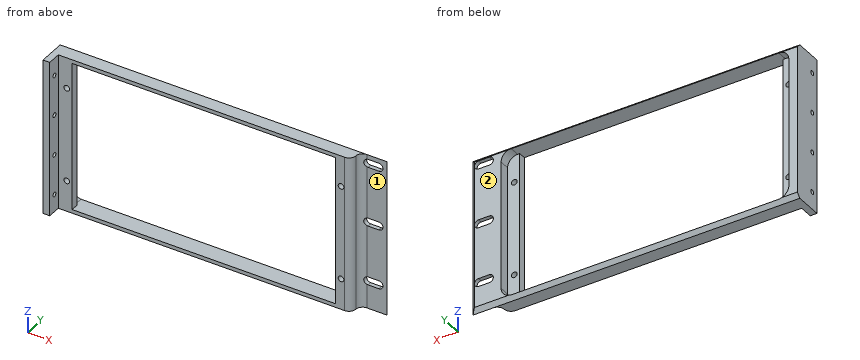
from build123d import *

# Parameters (mm, degrees)
SKETCH1_W                        = 242.5
SKETCH1_H                        = 116
BOSS_EXTRUDE1_DEPTH              = 13
CUT_EXTRUDE1_DEPTH               = 7.6
F_1_8_27_NPSM_TAPPED_HOLE1_D     = 5
F_1_8_27_NPSM_TAPPED_HOLE1_DEPTH = 22.99
F_1_8_27_NPSM_TAPPED_HOLE1_TIP   = 1.502151548
SKETCH6_W                        = 195.5
SKETCH6_H                        = 110.5
CUT_EXTRUDE2_DEPTH               = 143.098592533
SKETCH32_W                       = 20
SKETCH32_H                       = 116
CUT_EXTRUDE10_DEPTH              = 10
FILLET1_START                    = -59
FILLET1_DEPTH                    = 118
FILLET1_START_2                  = -58
FILLET1_2_DEPTH                  = 116
CHAMFER1_SIZE                    = 3
SKETCH36_W                       = 5
SKETCH36_H                       = 116
BOSS_EXTRUDE2_DEPTH              = 10
M5X0_8_TAPPED_HOLE1_D            = 4.2
M5X0_8_TAPPED_HOLE1_DEPTH        = 12.4
M5X0_8_TAPPED_HOLE1_TIP          = 1.2618073
M4X0_7_TAPPED_HOLE1_D            = 3.3
CUT_EXTRUDE11_DEPTH              = 144.747173885


with BuildPart() as part:
    # Sketch1 → Boss-Extrude1 (new body)
    with BuildSketch(Plane(origin=(0, 0, 0), x_dir=(1, 0, 0), z_dir=(0, 1, 0))):
        with Locations((8.25, 0)):
            Rectangle(SKETCH1_W, SKETCH1_H)
    extrude(amount=BOSS_EXTRUDE1_DEPTH)

    # Sketch2 → Cut-Extrude1 (cut)
    with BuildSketch(Plane(origin=(0, 13, 0), x_dir=(1, 0, 0), z_dir=(0, 1, 0))):
        with BuildLine():
            Line((-99.25, 55.25), (99.25, 55.25))
            ThreePointArc((99.25, 55.25), (104.553300859, 53.053300859), (106.75, 47.75))
            Line((106.75, 47.75), (106.75, -47.75))
            ThreePointArc((106.75, -47.75), (104.553300859, -53.053300859), (99.25, -55.25))
            Line((99.25, -55.25), (-99.25, -55.25))
            ThreePointArc((-99.25, -55.25), (-104.553300859, -53.053300859), (-106.75, -47.75))
            Line((-106.75, -47.75), (-106.75, 47.75))
            ThreePointArc((-106.75, 47.75), (-104.553300859, 53.053300859), (-99.25, 55.25))
        make_face()
    extrude(amount=-CUT_EXTRUDE1_DEPTH, mode=Mode.SUBTRACT)

    # 1/8-27 NPSM Tapped Hole1
    with Locations(Plane(origin=(0, 5.4, 0), x_dir=(1, 0, 0), z_dir=(0, 1, 0))):
        with Locations((-74.86, 30.93), (51.34, 30.93), (51.34, -34.72), (-74.86, -34.72)):
            Hole(F_1_8_27_NPSM_TAPPED_HOLE1_D / 2, depth=F_1_8_27_NPSM_TAPPED_HOLE1_DEPTH)
            with Locations((0, 0, -(F_1_8_27_NPSM_TAPPED_HOLE1_DEPTH + F_1_8_27_NPSM_TAPPED_HOLE1_TIP / 2))):  # 118° drill point
                Cone(0, F_1_8_27_NPSM_TAPPED_HOLE1_D / 2, F_1_8_27_NPSM_TAPPED_HOLE1_TIP, mode=Mode.SUBTRACT)

    # Sketch6 → Cut-Extrude2 (cut, through all)
    with BuildSketch(Plane(origin=(0, 5.4, 0), x_dir=(1, 0, 0), z_dir=(0, 1, 0))):
        Rectangle(SKETCH6_W, SKETCH6_H)
    extrude(amount=-CUT_EXTRUDE2_DEPTH, mode=Mode.SUBTRACT)

    # Sketch32 → Cut-Extrude10 (cut)
    with BuildSketch(Plane.XZ):
        with Locations((119.5, 0)):
            Rectangle(SKETCH32_W, SKETCH32_H)
    extrude(amount=-CUT_EXTRUDE10_DEPTH, mode=Mode.SUBTRACT)

    # Fillet1: read off the stored shape, not the designer's step
    # Fillet1 outline → Fillet1 (cut)
    with BuildSketch(Plane.XY.offset(FILLET1_START)):
        with BuildLine():
            Line((109.5, 0), (109.5, 5))
            ThreePointArc((109.5, 5), (108.035533906, 1.464466094), (104.5, 0))
            Line((104.5, 0), (109.5, 0))
        make_face()
    extrude(amount=FILLET1_DEPTH, mode=Mode.SUBTRACT)

    # Fillet1 2 outline → Fillet1 2 (add)
    with BuildSketch(Plane.XY.offset(FILLET1_START_2)):
        with BuildLine():
            ThreePointArc((109.5, 5), (110.964466094, 8.535533906), (114.5, 10))
            Line((114.5, 10), (109.5, 10))
            Line((109.5, 10), (109.5, 5))
        make_face()
    extrude(amount=FILLET1_2_DEPTH)

    # Chamfer1
    # the kernel refuses this chamfer: 3 mm, written as the material it takes off along each edge
    with BuildSketch(Plane(origin=(137.215048964, 13, 58), x_dir=(0, 0, -1), z_dir=(-1, 0, 0))) as chamfer1_piece_1:
        Polygon((CHAMFER1_SIZE, 0), (0, CHAMFER1_SIZE), (0, 0), align=None)
    extrude(amount=257.930097928, mode=Mode.SUBTRACT)
    with BuildSketch(Plane(origin=(129.5, 13, -65.715048964), x_dir=(0, -1, 0), z_dir=(0, 0, 1))) as chamfer1_piece_2:
        Polygon((CHAMFER1_SIZE, 0), (0, -CHAMFER1_SIZE), (0, 0), align=None)
    extrude(amount=131.430097928, mode=Mode.SUBTRACT)
    with BuildSketch(Plane(origin=(-120.715048964, 13, -58), x_dir=(0, -1, 0), z_dir=(1, 0, 0))) as chamfer1_piece_3:
        Polygon((CHAMFER1_SIZE, 0), (0, -CHAMFER1_SIZE), (0, 0), align=None)
    extrude(amount=257.930097928, mode=Mode.SUBTRACT)

    # Sketch36 → Boss-Extrude2 (add)
    with BuildSketch(Plane.XZ):
        with Locations((-110.5, 0)):
            Rectangle(SKETCH36_W, SKETCH36_H)
    extrude(amount=BOSS_EXTRUDE2_DEPTH)

    # M5x0.8 Tapped Hole1
    with Locations(Plane(origin=(0, 5.4, 0), x_dir=(1, 0, 0), z_dir=(0, 1, 0))):
        with Locations((-101.75, 35), (-101.75, -35), (101.75, 35), (101.75, -35)):
            Hole(M5X0_8_TAPPED_HOLE1_D / 2, depth=M5X0_8_TAPPED_HOLE1_DEPTH)
            with Locations((0, 0, -(M5X0_8_TAPPED_HOLE1_DEPTH + M5X0_8_TAPPED_HOLE1_TIP / 2))):  # 118° drill point
                Cone(0, M5X0_8_TAPPED_HOLE1_D / 2, M5X0_8_TAPPED_HOLE1_TIP, mode=Mode.SUBTRACT)

    # M4x0.7 Tapped Hole1 (through all)
    with Locations(Plane(origin=(-108, 0, 0), x_dir=(0, 0, -1), z_dir=(1, 0, 0))):
        with Locations((-15, -4.5), (15, -4.5), (45, -4.5), (-45, -4.5)):
            Hole(M4X0_7_TAPPED_HOLE1_D / 2)

    # Sketch43 → Cut-Extrude11 (cut, through all)
    with BuildSketch(Plane(origin=(0, 13, 0), x_dir=(1, 0, 0), z_dir=(0, 1, 0))):
        with BuildLine():
            Line((115.5, -48.65), (123.5, -48.65))
            ThreePointArc((123.5, -48.65), (126.5, -51.65), (123.5, -54.65))
            Line((123.5, -54.65), (115.5, -54.65))
            ThreePointArc((115.5, -54.65), (112.5, -51.65), (115.5, -48.65))
        make_face()
        with BuildLine():
            Line((115.5, -4.2), (123.5, -4.2))
            ThreePointArc((123.5, -4.2), (126.5, -7.2), (123.5, -10.2))
            Line((123.5, -10.2), (115.5, -10.2))
            ThreePointArc((115.5, -10.2), (112.5, -7.2), (115.5, -4.2))
        make_face()
        with BuildLine():
            Line((115.5, 40.25), (123.5, 40.25))
            ThreePointArc((123.5, 40.25), (126.5, 37.25), (123.5, 34.25))
            Line((123.5, 34.25), (115.5, 34.25))
            ThreePointArc((115.5, 34.25), (112.5, 37.25), (115.5, 40.25))
        make_face()
    extrude(amount=-CUT_EXTRUDE11_DEPTH, mode=Mode.SUBTRACT)


solid = part.part
Here's how the part is built. I have some questions about the finished solid (model axes, mm). Face numbers are marked on the shaded views. A direction names the side the tool comes from. Round coordinates to 2 decimals unless told otherwise and drop trailing zeros. Loops run counter-clockwise (first coordinate to the right, second up) from the corner with the lowest first, then second, coordinate; pieces in that order, holes last. Notation, with made-up numbers: M 84,54.25 L 122,54.25 A27 cw 122,90.25 Z; hole C -16.5,57 d7. An arc over 180 degrees is marked long. Write each question's results on one line, items separated by ' | '. Start each with the question number.
(1) I want a section at A-A (x = 5.5). Please give me the cut outline in (y, z).
(2) If I drill on probe 1 along X at (y, z) = (4.35, -35); probe 2 along Z at (x, y) = (-77, 4.25); probe 3 along X at (y, z) = (3.4, -35), over which ranges is the centre line in solid material (lowest first)? Write a range as from..to.
(3) On a 3-axis mill with a long thin cutter (end or side, diameter ignored), from which of +Z, -Z, +X, -X, +Y, -Y can I reach the whole of each face in a straight line? I mean the marked faces 1 and 2. Say none if no direction works.
(4) Will these pins go through, and if not, where does the flat tip stop? P1, Ø12, axis at x = 121, z = -27.5, coming from the -Y side; P2, Ø0.9, axis at x = 121.5, y = 11, coming from the +Z side; P3, Ø0.9, axis at x = 119.5, y = 11, coming from the -Z side.
Solved:
1) outline: M 0,-58 L 10,-58 L 12.75,-55.25 L 0,-55.25 Z; M 0,55.25 L 12.75,55.25 L 10,58 L 0,58 Z
2) probe 1: x = -113..-103.85, -99.65..-97.75, 97.75..99.65, 103.85..109.46 | probe 2: z = -58..-55.25, 55.25..58 | probe 3: x = -113..-103.85, -99.65..-97.75, 97.75..99.65, 103.85..109.24
3) face 1: +Z, -Z, +X, -Y | face 2: +Z, -Z, +X, -X, +Y
4) P1: stops at y = 10 | P2: stops at z = 57.45 | P3: stops at z = -57.45
